```python
from build123d import *

# Parameters (mm, degrees)
F2_R = 0.3
F3_R = 0.3
F4_R = 0.3


with BuildPart() as f1:
    # F0 (on Right) → F1 (revolve)
    with BuildSketch(Plane.YZ):
        Polygon((1.9, 61.867032), (0, 61.867032), (0, 60.867032), (1.7, 60.867032), (1.7, 52.617032), (8.325, 52.617032), (8.325, 53.867032), (1.9, 53.867032), align=None)
    revolve(axis=Axis((0, 0, 61.367032), (0, 0, 1)))

    # F2
    f2_edges = [f1.edges().sort_by_distance(p)[0] for p in [
        (0, -1.9, 61.867032),
    ]]
    fillet(f2_edges, radius=F2_R)

    # F3
    f3_edges = [f1.edges().sort_by_distance(p)[0] for p in [
        (0, -8.325, 53.867032),
    ]]
    fillet(f3_edges, radius=F3_R)

    # F4
    f4_edges = [f1.edges().sort_by_distance(p)[0] for p in [
        (0, -1.9, 53.867032),
    ]]
    fillet(f4_edges, radius=F4_R)


solid = f1.part
```
For this review, take the finished solid that the model builds, in its own axes (mm). A direction names the side the tool comes from. Round coordinates to 2 decimals unless told otherwise and drop trailing zeros. Loops run counter-clockwise (first coordinate to the right, second up) from the corner with the lowest first, then second, coordinate; pieces in that order, holes last.
(1) We need section C-C (z = 54.5). Give the boundary of the cut face in (x, y), plus the area to 3 significant figures.
Returned:
outline: circle Ø3.8 at (0, 0); hole circle Ø3.4 at (0, 0)
area: 2.26 mm2
(2) Wall thickness on line 1 along Y through (x, z) = (0, 57.5); line 2 along Z through (x, y) = (-1, -0.75): over which ranges is each line inside the solid? List them lowest first.
Returned:
line 1: y = -1.9 to -1.7, 1.7 to 1.9
line 2: z = 60.87 to 61.87
(3) Tool access review of faces 5 (the flat face through (2, 0, 52.617)), 6 (the flat face through (2, 2, 53.867)): name each direction out of +Z, -Z, +X, -X, +Y, -Y from which nothing blocks a thin tool from reaching the whole face with its end or side.
Returned:
face 5: -Z, +X, -X, +Y, -Y
face 6: +Z
(4) Mouldability with a two-part tool opening along X and no side actions: class faces 1 (the cylindrical face through (7.386, 3.841, 53.099)), 2 (the flat face through (0, 0, 60.867)), 3 (the cylindrical face through (1.66, -0.37, 56.68)), 4 (the flat face through (0, 0, 61.867)) as released by +X, released by -X, zero draft, split by the parting line, or undercut.
Returned:
face 1: split by the parting line
face 2: undercut
face 3: undercut
face 4: zero draft
(5) We need section A-A (x = 0). Give the boundary of the cut face in (y, z) (3 decimals).
Returned:
outline: (-8.325, 52.617) - (-1.7, 52.617) - (-1.7, 60.867) - (1.7, 60.867) - (1.7, 52.617) - (8.325, 52.617) - (8.325, 53.567) arc R0.3 ccw to (8.025, 53.867) - (2.2, 53.867) arc R0.3 cw to (1.9, 54.167) - (1.9, 61.567) arc R0.3 ccw to (1.6, 61.867) - (-1.6, 61.867) arc R0.3 ccw to (-1.9, 61.567) - (-1.9, 54.167) arc R0.3 cw to (-2.2, 53.867) - (-8.025, 53.867) arc R0.3 ccw to (-8.325, 53.567) - close
(6) Clearance check with flat-ended pins moving along their axes: P1, Ø2.5, axis at x = 0, y = 0, coming from the -Z side; P2, Ø4, axis at x = 4.5, z = 60.5, coming from the +Y side; P3, Ø2, axis at x = 4.5, z = 54.5, coming from the +Y side; P4, Ø5, axis at x = -5.5, z = 54, coming from the +Y side. State where each tip first meets the part, or that it passes through.
Returned:
P1: stops at z = 60.87
P2: passes through
P3: stops at y = 7.32
P4: stops at y = 7.75
